```python
from build123d import *

# Parameters (mm, degrees)
SKETCH1_R           = 3.75
BOSS_EXTRUDE1_DEPTH = 30
SKETCH2_R           = 3.75
BOSS_EXTRUDE2_DEPTH = 30
CUT_EXTRUDE1_DEPTH  = 29.0000001
SKETCH4_W           = 5.792740578
SKETCH4_H           = 11.5
BOSS_EXTRUDE3_DEPTH = 10
BOSS_EXTRUDE4_DEPTH = 10
SKETCH5_R           = 2.5
CUT_EXTRUDE2_DEPTH  = 31.0000001
SKETCH7_R           = 3.75
CUT_EXTRUDE3_DEPTH  = 31.155444666
SKETCH8_R           = 3.75
CUT_EXTRUDE4_DEPTH  = 38.57772242


with BuildPart() as part:
    # Sketch1 → Boss-Extrude1 (new body)
    with BuildSketch(Plane(origin=(0, 0, 0), x_dir=(0, 0, -1), z_dir=(1, 0, 0))):
        with BuildLine():
            Line((-8.75, 0), (8.75, 0))
            Line((8.75, 0), (8.75, 10.75))
            ThreePointArc((8.75, 10.75), (0, 19.5), (-8.75, 10.75))
            Line((-8.75, 10.75), (-8.75, 0))
        make_face()
        with Locations((0, 10.75)):
            Circle(SKETCH1_R, mode=Mode.SUBTRACT)
    extrude(amount=BOSS_EXTRUDE1_DEPTH)

    # Sketch2 → Boss-Extrude2 (add)
    with BuildSketch(Plane(origin=(-3.788861142, 0, 6.5625), x_dir=(-0.866025404, 0, -0.5), z_dir=(0.5, 0, -0.866025404))):
        with BuildLine():
            Line((-4.375, 0), (-4.375, 19.25))
            ThreePointArc((-4.375, 19.25), (-13.125, 28), (-21.875, 19.25))
            Line((-21.875, 19.25), (-21.875, 0))
            Line((-21.875, 0), (-4.375, 0))
        make_face()
        with Locations((-13.125, 19.25)):
            Circle(SKETCH2_R, mode=Mode.SUBTRACT)
    extrude(amount=BOSS_EXTRUDE2_DEPTH)

    # Sketch3 → Cut-Extrude1 (cut, through all)
    with BuildSketch(Plane.XZ):
        with BuildLine():
            Line((24.207259422, 8.75), (24.207259422, 15.67820323))
            Line((24.207259422, 15.67820323), (16.207259422, 15.67820323))
            Line((16.207259422, 15.67820323), (16.207259422, 8.75))
            ThreePointArc((16.207259422, 8.75), (20.207259422, 4.75), (24.207259422, 8.75))
        make_face()
    extrude(amount=-CUT_EXTRUDE1_DEPTH, mode=Mode.SUBTRACT)

    # Sketch4 → Boss-Extrude3 (add)
    with BuildSketch(Plane.XZ):
        with Locations((27.103629711, 14.5)):
            Rectangle(SKETCH4_W, SKETCH4_H)
    extrude(amount=-BOSS_EXTRUDE3_DEPTH)

    # Sketch6 → Boss-Extrude4 (add)
    with BuildSketch(Plane.XZ):
        Polygon((16.207259422, 15.67820323), (16.207259422, 20.25), (9.526279442, 20.25), (9.526279442, 14.25), align=None)
    extrude(amount=-BOSS_EXTRUDE4_DEPTH)

    # Sketch5 → Cut-Extrude2 (cut, through all)
    with BuildSketch(Plane(origin=(30, 0, 0), x_dir=(0, 0, -1), z_dir=(1, 0, 0))):
        with Locations(Location((-15.25, 5, 0), (0, 0, 66.421821522))):  # turned: the seam where the file's is
            Circle(SKETCH5_R)
    extrude(amount=-CUT_EXTRUDE2_DEPTH, mode=Mode.SUBTRACT)

    # Sketch7 → Cut-Extrude3 (cut, through all)
    with BuildSketch(Plane.ZY):
        with Locations(Location((0, 10.75, 0), (0, 0, 180))):  # turned: the seam where the file's is
            Circle(SKETCH7_R)
    extrude(amount=-CUT_EXTRUDE3_DEPTH, mode=Mode.SUBTRACT)

    # Sketch8 → Cut-Extrude4 (cut, through all)
    with BuildSketch(Plane(origin=(-3.788861142, 0, 6.5625), x_dir=(0.866025404, 0, 0.5), z_dir=(-0.5, 0, 0.866025404))):
        with Locations(Location((13.125, 19.25, 0), (0, 0, 180))):  # turned: the seam where the file's is
            Circle(SKETCH8_R)
    extrude(amount=-CUT_EXTRUDE4_DEPTH, mode=Mode.SUBTRACT)


with BuildPart() as body_2:
    # Mirror1: mirrored copy
    add(part.part.mirror(Plane(origin=(30, 0, 8.75), x_dir=(0, 0, 1), z_dir=(0, 1, 0))))


solid = body_2.part
```
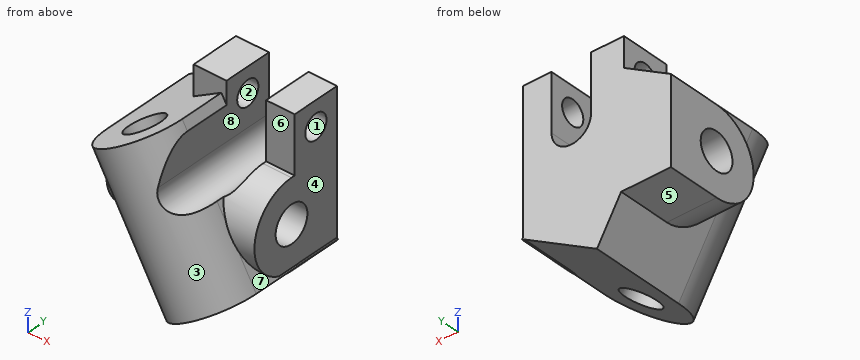
CAD build for the part. Positions are in the model's coordinates, mm. Face numbers are marked on the shaded views. A direction names the side the tool comes from. Give positions to 0.01 mm unless a question says otherwise; leave off trailing zeros. Loops run counter-clockwise (first coordinate to the right, second up) from the corner with the lowest first, then second, coordinate; pieces in that order, holes last. Notation, with made-up numbers: (8, 65) -> (47, 65) arc R4 cw to (47, 71) -> close; hole circle Ø6 at (68, 15.25). An arc over 180 degrees is marked (long way). Use a Markdown table: item, result.
1. Slice it at C-C (z = 3). Give the number of separate pieces and of enclosed holes in the cut face, plus the area to 3 significant figures.
Check result:
| item | result |
|---|---|
| separate pieces | 2 |
| enclosed holes | 1 |
| area | 528 mm^2 |
2. Wall check: L1, parallel to Y at x = 26.45, z = 15.25; L2, parallel to Y at x = 13.5, z = 0; L3, parallel to X at y = -20, z = -6. Give the ranges that are in metal, low to high. Write a range as [from, to].
Check result:
| item | result |
|---|---|
| L1 | y = [-10, -7.5], [-2.5, 0] |
| L2 | y = [-27.88, -22.72], [-15.78, -14.5], [-7, 0] |
| L3 | x = [8.55, 14.38], [22.86, 28.69] |
3. Which spindle directions (+Z, -Z, +X, -X, +Y, -Y) get a long thin tool onto all of the face, cutting with end or side? Do the marked faces 5, 6, 7 and 8. Say none if no direction does.
Check result:
| item | result |
|---|---|
| face 5 | -Z, -X, +Y, -Y |
| face 6 | +Z, +X, -Y |
| face 7 | +X, -Y |
| face 8 | +Z, +Y, -Y |
4. Slice it at B-B (y = -4.5). List the corners of the cut face in (x, z).
Check result:
| item | result |
|---|---|
| outline | (0, -8.75) -> (10.1, -8.75) -> (15, -17.23) -> (29.69, -8.75) -> (30, -8.75) -> (30, -8.57) -> (30.16, -8.48) -> (30, -8.21) -> (30, 12.8) -> (24.21, 12.8) -> (24.21, 8.75) arc R4 cw to (16.21, 8.75) -> (16.21, 12.8) -> (7.02, 12.8) -> (0, 8.75) -> close; (9.53, 17.7) -> (16.21, 17.7) -> (16.21, 20.25) -> (9.53, 20.25) -> close; (24.21, 17.7) -> (30, 17.7) -> (30, 20.25) -> (24.21, 20.25) -> close |
5. Flat gauge pins, fed straight in: pin 1 (0.8 mm diameter, centred on x = 27, y = -10.5, fed in from +Z); pin 2 (12 mm diameter, centred on y = -10.75, z = 0, fed in from +X); pin 3 (1.8 mm diameter, centred on x = 14, z = 16, fed in from -Y). Where does each tip first touch, or does it go through?
Check result:
| item | result |
|---|---|
| pin 1 | stops at z = 8.75 |
| pin 2 | stops at x = 30 |
| pin 3 | stops at y = -25.52 |
6. Slice it at D-D (y = -25.5). List the corners of the cut face in (x, z).
Check result:
| item | result |
|---|---|
| outline | (2.27, 10.06) -> (17.27, -15.92) -> (27.88, -9.79) -> (19.44, 4.82) arc R4 cw to (16.21, 8.75) -> (16.21, 10.43) -> (12.88, 16.19) -> close |
7. Slice it at A-A (y = -20.5). List the corners of the cut face in (x, z).
Check result:
| item | result |
|---|---|
| outline | (0.08, 8.79) -> (15.08, -17.19) -> (19.52, -14.62) -> (4.52, 11.36) -> close; (10.64, 14.89) -> (25.64, -11.09) -> (30.08, -8.53) -> (22.13, 5.24) arc R4 cw to (16.21, 8.75) -> (16.21, 15.5) -> (15.08, 17.46) -> close |
8. Mould opens along Y. For the marked faces 1, 2, 3 and 4 say: pulls with the +Y half, pulls with the -Y half, needs draft (parallel to the pull), parting line crosses it, or undercut.
Check result:
| item | result |
|---|---|
| face 1 | undercut |
| face 2 | undercut |
| face 3 | pulls with the -Y half |
| face 4 | needs draft |
